CAD build for the part. Positions are in the model's coordinates, mm. Coordinates: 2 decimals unless noted, no trailing zeros. Loops run counter-clockwise (first coordinate to the right, second up) from the corner with the lowest first, then second, coordinate; pieces in that order, holes last. Notation, with made-up numbers: (59, 18) - (90, 18) arc R12 cw to (90, 36) - close; hole circle Ø3 at (88.5, -22). An arc over 180 degrees is marked (long way). Put each result on its own line as item: value.
```python
from build123d import *

# Parameters (mm, degrees)
SKETCH5_R               = 12.7
SKETCH5_R_2             = 7.9375
BOSS_EXTRUDE2_DEPTH     = 3.175
SKETCH8_W               = 6.35
SKETCH8_H               = 6.35
CUT_EXTRUDE1_DEPTH      = 4.175
CUT_EXTRUDE1_DEPTH_BACK = 4.175
SKETCH9_R               = 6.35
CUT_EXTRUDE2_DEPTH      = 4.175
CUT_EXTRUDE2_DEPTH_BACK = 4.175


with BuildPart() as part:
    # Sketch5 → Boss-Extrude2 (new body, symmetric)
    with BuildSketch(Plane.XY):
        with BuildLine():
            Line((-223.779910529, -44.577802506), (-54.04268144, -3.827499177))
            ThreePointArc((-54.04268144, -3.827499177), (-42.924981025, 2.041131203), (-35.983316209, 12.522418081))
            ThreePointArc((-35.983316209, 12.522418081), (0, 38.1), (35.983316209, 12.522418081))
            ThreePointArc((35.983316209, 12.522418081), (42.924981025, 2.041131203), (54.04268144, -3.827499177))
            Line((54.04268144, -3.827499177), (223.779910529, -44.577802506))
            ThreePointArc((223.779910529, -44.577802506), (239.972758508, -56.795566669), (242.055998097, -76.973331649))
            ThreePointArc((242.055998097, -76.973331649), (0, -254), (-242.055998097, -76.973331649))
            ThreePointArc((-242.055998097, -76.973331649), (-239.972758508, -56.795566669), (-223.779910529, -44.577802506))
        make_face()
        Circle(SKETCH5_R, mode=Mode.SUBTRACT)
        with Locations((-117.332700629, -48.60079591)):
            Circle(SKETCH5_R_2, mode=Mode.SUBTRACT)
        with Locations((117.332700629, -48.60079591)):
            Circle(SKETCH5_R_2, mode=Mode.SUBTRACT)
    extrude(amount=BOSS_EXTRUDE2_DEPTH, both=True)

    # Sketch8 → Cut-Extrude1 (cut, two sides)
    with BuildSketch(Plane.XY) as cut_extrude1_sk:
        with Locations((0, 12.7)):
            Rectangle(SKETCH8_W, SKETCH8_H)
    extrude(amount=CUT_EXTRUDE1_DEPTH, mode=Mode.SUBTRACT)
    extrude(cut_extrude1_sk.sketch, amount=-CUT_EXTRUDE1_DEPTH_BACK, mode=Mode.SUBTRACT)

    # Sketch9 → Cut-Extrude2 (cut, two sides)
    with BuildSketch(Plane.XY) as cut_extrude2_sk:
        with Locations((0, -63.5)):
            Circle(SKETCH9_R)
        with Locations((0, -190.5)):
            Circle(SKETCH9_R)
    extrude(amount=CUT_EXTRUDE2_DEPTH, mode=Mode.SUBTRACT)
    extrude(cut_extrude2_sk.sketch, amount=-CUT_EXTRUDE2_DEPTH_BACK, mode=Mode.SUBTRACT)


solid = part.part
```
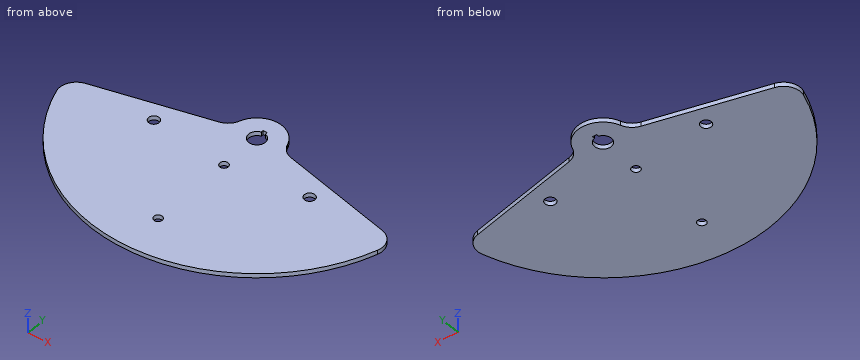
Q1. Slice it at B-B, the plane z = 1.5. State how many separate pieces and enclosed holes the cut face has, then the cut area to 3 significant figures.
Determined:
separate pieces: 1
enclosed holes: 5
area: 91,200 mm2
Q2. Slice it at C-C, the plane y = -63.5. Give the cut face in (x, z) (3 decimals), then the cut area to 3 significant figures.
Determined:
outline: (-242.585, -3.175) - (-6.35, -3.175) - (-6.35, 3.175) - (-242.585, 3.175) - close; (6.35, -3.175) - (242.585, -3.175) - (242.585, 3.175) - (6.35, 3.175) - close
area: 3,000 mm2
Q3. Pin check, flat tips, straight feed: pin 1 Ø15 at (x, y) = (0, 0) entering from +Z; pin 2 Ø1.5 at (x, z) = (165.5, -1.5) entering from +Y; pin 3 Ø1.5 at (y, z) = (-192.5, -0.5) entering from +X; pin 4 Ø1.8 at (y, z) = (14, -1) entering from -X. Stop position of each tip, or through.
Determined:
pin 1: through
pin 2: y = -30.41
pin 3: x = 166.58
pin 4: x = -35.78
Q4. Wall check: L1, parallel to Y at x = 0, z = -1.5 (3 decimals); L2, parallel to X at y = -63.5, z = 0.25; L3, parallel to Y at x = 114.5, z = -2.25. Give the ranges that are in metal, low to high. Write a range as from..to.
Determined:
L1: -254..-196.85, -184.15..-69.85, -57.15..-12.7, 15.875..38.1
L2: -242.58..-6.35, 6.35..242.58
L3: -226.73..-56.02, -41.19..-18.34
Q5. Slice it at A-A, the plane y = -190.5. Give the cut face in (x, z) (3 decimals), then the cut area to 3 significant figures.
Determined:
outline: (-168.005, -3.175) - (-6.35, -3.175) - (-6.35, 3.175) - (-168.005, 3.175) - close; (6.35, -3.175) - (168.005, -3.175) - (168.005, 3.175) - (6.35, 3.175) - close
area: 2,050 mm2
Q6. Slice it at D-D, the plane x = 151. Give the cut face in (y, z) (1 decimal), then the cut area to 3 significant figures.
Determined:
outline: (-204.2, -3.2) - (-27.1, -3.2) - (-27.1, 3.2) - (-204.2, 3.2) - close
area: 1,120 mm2
